Geometry check sheet. Reference: the model listing, model coordinates, mm. Face numbers are marked on the shaded views. A direction names the side the tool comes from. Round coordinates to 2 decimals unless told otherwise and drop trailing zeros. Order: outer loops, then holes, each group sorted by start corner. A loop starts at its lowest first (then second) coordinate and runs counter-clockwise, first axis right, second up.
(1) Release check for a two-part mould opening along X. For the marked faces 4, 5 and 6 record: +X half, -X half, draft (parallel to the pull), parting line (faces both ways), or undercut.
(2) Sectioned sample at C-C (x = 28). Record the boundary of the cut face in (y, z), plus the area to 3 significant figures.
(3) Go/stop test with flat-tipped pins: pin 1 (6.5 mm diameter, centred on x = -3.31, z = 10.66, fed in from +Y); pin 2 (4.5 mm diameter, centred on x = 47.69, z = 17.16, fed in from -Y). Record where each tip stops, or that it passes through.
(4) Set-up check for the marked faces 1, 2 and 3: record each of +Z, -Z, +X, -X, +Y, -Y from which the full face is reachable in a straight line by a thin tool's end or side.
(5) Sectioned sample at D-D (y = -3). Give the number of separate pieces and of enclosed holes in the cut face, plus the area to 3 significant figures.
(6) Material ranges on line 1 along X through (y, z) = (-3.25, 11); line 2 along X through (y, z) = (-2.5, 9.75); line 3 along Z through (x, y) = (30, -3.25), recorded low to high.
(7) Sectioned sample at A-A (x = 0.5). Record the boundary of the cut face in (y, z), plus the area to 3 significant figures.
(8) Sectioned sample at B-B (z = 20). Record the boundary of the cut face in (x, y), plus the area to 3 significant figures.
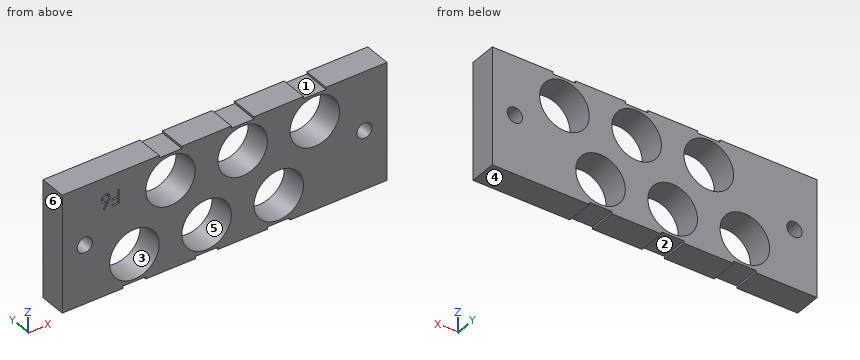
from build123d import *

# Parameters (mm, degrees)
SKETCH1_R               = 5.5
BOSS_EXTRUDE1_DEPTH     = 6
BOSS_EXTRUDE1_2_DEPTH   = 6
BOSS_EXTRUDE1_3_DEPTH   = 6
BOSS_EXTRUDE1_4_DEPTH   = 6
BOSS_EXTRUDE1_5_DEPTH   = 6
BOSS_EXTRUDE1_6_DEPTH   = 6
BOSS_EXTRUDE2_START     = -6
BOSS_EXTRUDE2_OUTLINE_R = 1.7
BOSS_EXTRUDE2_DEPTH     = 6
CUT_EXTRUDE1_DEPTH      = 1


# Read off the part's stored shape, not the designer's step: Boss-Extrude2
with BuildPart() as part:
    # Sketch1 → Boss-Extrude1 (new body)
    with BuildSketch(Plane(origin=(0, 0, 0), x_dir=(1, 0, 0), z_dir=(0, 1, 0))):
        Polygon((2.686395113, -16.66487452), (2.68639507, -4.66487452), (-9.31360493, -4.664874562), (-9.313604887, -16.664874562), align=None)
        with Locations(Location((-3.313604908, -10.664874541, 0), (0, 0, 270))):
            Circle(SKETCH1_R, mode=Mode.SUBTRACT)
    extrude(amount=-BOSS_EXTRUDE1_DEPTH)



with BuildPart() as body_2:
    # Sketch1 → Boss-Extrude1 2 (new body)
    with BuildSketch(Plane(origin=(0, 0, 0), x_dir=(1, 0, 0), z_dir=(0, 1, 0))):
        Polygon((18.686395113, -16.664873819), (18.68639507, -4.664873819), (6.68639507, -4.664873862), (6.686395113, -16.664873862), align=None)
        with Locations(Location((12.686395092, -10.66487384, 0), (0, 0, 270))):
            Circle(SKETCH1_R, mode=Mode.SUBTRACT)
    extrude(amount=-BOSS_EXTRUDE1_2_DEPTH)


with BuildPart() as body_3:
    # Sketch1 → Boss-Extrude1 3 (new body)
    with BuildSketch(Plane(origin=(0, 0, 0), x_dir=(1, 0, 0), z_dir=(0, 1, 0))):
        Polygon((34.686395113, -16.664873762), (34.68639507, -4.664873762), (22.68639507, -4.664873805), (22.686395113, -16.664873805), align=None)
        with Locations(Location((28.686395092, -10.664873784, 0), (0, 0, 270))):
            Circle(SKETCH1_R, mode=Mode.SUBTRACT)
    extrude(amount=-BOSS_EXTRUDE1_3_DEPTH)


with BuildPart() as body_4:
    # Sketch1 → Boss-Extrude1 4 (new body)
    with BuildSketch(Plane(origin=(0, 0, 0), x_dir=(1, 0, 0), z_dir=(0, 1, 0))):
        Polygon((14.68639512, -17.664873833), (14.686395163, -29.664873833), (26.686395163, -29.664873791), (26.68639512, -17.664873791), align=None)
        with Locations(Location((20.686395141, -23.664873812, 0), (0, 0, 270))):
            Circle(SKETCH1_R, mode=Mode.SUBTRACT)
    extrude(amount=-BOSS_EXTRUDE1_4_DEPTH)


with BuildPart() as body_5:
    # Sketch1 → Boss-Extrude1 5 (new body)
    with BuildSketch(Plane(origin=(0, 0, 0), x_dir=(1, 0, 0), z_dir=(0, 1, 0))):
        Polygon((-1.31360488, -17.664873456), (-1.313604837, -29.664873456), (10.686395163, -29.664873413), (10.68639512, -17.664873413), align=None)
        with Locations(Location((4.686395141, -23.664873434, 0), (0, 0, 270))):
            Circle(SKETCH1_R, mode=Mode.SUBTRACT)
    extrude(amount=-BOSS_EXTRUDE1_5_DEPTH)


with BuildPart() as body_6:
    # Sketch1 → Boss-Extrude1 6 (new body)
    with BuildSketch(Plane(origin=(0, 0, 0), x_dir=(1, 0, 0), z_dir=(0, 1, 0))):
        Polygon((30.68639512, -17.664873979), (30.686395163, -29.664873979), (42.686395163, -29.664873936), (42.68639512, -17.664873936), align=None)
        with Locations(Location((36.686395141, -23.664873958, 0), (0, 0, 270))):
            Circle(SKETCH1_R, mode=Mode.SUBTRACT)
    extrude(amount=-BOSS_EXTRUDE1_6_DEPTH)


with BuildPart() as part_1:
    add(part.part)

    add(body_2.part)  # Boss-Extrude2 merges body 2

    add(body_3.part)  # Boss-Extrude2 merges body 3

    add(body_4.part)  # Boss-Extrude2 merges body 4

    add(body_5.part)  # Boss-Extrude2 merges body 5

    add(body_6.part)  # Boss-Extrude2 merges body 6
    # Boss-Extrude2 outline → Boss-Extrude2 (add)
    with BuildSketch(Plane(origin=(0, 0, 0), x_dir=(1, 0, 0), z_dir=(0, 1, 0)).offset(BOSS_EXTRUDE2_START)):
        Polygon((10.186395069, -4.164873849), (-0.813604931, -4.164873888), (-0.81360493, -4.664874532), (2.68639507, -4.66487452), (2.686395113, -16.66487452), (-9.313604887, -16.664874562), (-9.31360493, -4.664874562), (-5.81360493, -4.66487455), (-5.813604931, -4.16487455), (-19.313604998, -4.164874546), (-19.313604998, -30.16487344), (2.186395164, -30.164873443), (2.186395163, -29.664873443), (-1.313604837, -29.664873456), (-1.31360488, -17.664873456), (10.68639512, -17.664873413), (10.686395163, -29.664873413), (7.186395163, -29.664873426), (7.186395164, -30.164873425), (18.186395164, -30.164873821), (18.186395163, -29.664873821), (14.686395163, -29.664873833), (14.68639512, -17.664873833), (26.68639512, -17.664873791), (26.686395163, -29.664873791), (23.186395163, -29.664873803), (23.186395164, -30.164873803), (34.186395164, -30.164873764), (34.186395163, -29.664873966), (30.686395163, -29.664873979), (30.68639512, -17.664873979), (42.68639512, -17.664873936), (42.686395163, -29.664873936), (39.186395163, -29.664873949), (39.186395164, -30.164873949), (52.686395098, -30.16487344), (52.686395098, -4.164874546), (31.186395069, -4.164873775), (31.18639507, -4.664873775), (34.68639507, -4.664873762), (34.686395113, -16.664873762), (22.686395113, -16.664873805), (22.68639507, -4.664873805), (26.18639507, -4.664873792), (26.186395069, -4.164873793), (15.186395069, -4.164873832), (15.18639507, -4.664873832), (18.68639507, -4.664873819), (18.686395113, -16.664873819), (6.686395113, -16.664873862), (6.68639507, -4.664873862), (10.18639507, -4.664873849), align=None)
        with Locations((-14.313604998, -17.164873993)):
            Circle(BOSS_EXTRUDE2_OUTLINE_R, mode=Mode.SUBTRACT)
        with Locations((47.686395098, -17.164873993)):
            Circle(BOSS_EXTRUDE2_OUTLINE_R, mode=Mode.SUBTRACT)
    extrude(amount=BOSS_EXTRUDE2_DEPTH)

    # Sketch2 → Cut-Extrude1 (cut)
    # profile 1 of 2: a face of its own
    with BuildSketch(Plane(origin=(0, -6, 0), x_dir=(-1, 0, 0), z_dir=(0, -1, 0))):
        Polygon((6.699801581, -23.2390136), (8.246596453, -23.2390136), (8.246596453, -23.564654626), (6.984737478, -23.564654626), (6.984737478, -24.541577703), (8.246596453, -24.541577703), (8.246596453, -24.867218728), (6.984737478, -24.867218728), (6.984737478, -26.4140136), (6.699801581, -26.4140136), align=None)
    # profile 2 of 2: a face of its own
    with BuildSketch(Plane(origin=(0, -6, 0), x_dir=(-1, 0, 0), z_dir=(0, -1, 0))):
        with BuildLine():
            Line((9.996916965, -23.157603344), (10.216979065, -23.329964121))
            Line((10.216979065, -23.329964121), (9.378071813, -24.612811677))
            add(Edge.make_bspline(
                [(9.378071813, -24.612811677), (9.43392485, -24.603909103), (9.542872514, -24.586543627), (9.65315015, -24.583678919), (9.706892927, -24.582282831)],
                knots=[0, 0, 0, 0, 1.025318673, 2, 2, 2, 2], degree=3))
            add(Edge.make_bspline(
                [(9.706892927, -24.582282831), (9.739163887, -24.583137599), (9.802478203, -24.584814619), (9.895509725, -24.598067595), (9.984924431, -24.618695779), (10.070522851, -24.64888638), (10.152413619, -24.68743998), (10.231065003, -24.733649384), (10.30499899, -24.789897237), (10.375167554, -24.852730491), (10.438873565, -24.922323744), (10.49527613, -24.996166388), (10.542653291, -25.074181472), (10.581092491, -25.156329486), (10.610941917, -25.2424838), (10.632702138, -25.332534184), (10.645565054, -25.426542733), (10.647311749, -25.490476506), (10.648199017, -25.522952903)],
                knots=[0, 0, 0, 0, 1.044136307, 2.048553127, 3.035567123, 4.010001674, 4.980053131, 5.96154148, 6.956538004, 7.981742224, 9.006487041, 10.005615874, 10.984750588, 11.954802044, 12.935714515, 13.930994945, 14.949008866, 16, 16, 16, 16], degree=3))
            add(Edge.make_bspline(
                [(10.648199017, -25.522952903), (10.646908057, -25.567384491), (10.644367755, -25.654815343), (10.619055025, -25.782157069), (10.579721633, -25.903471565), (10.523499161, -26.016821942), (10.453665142, -26.122052845), (10.368504755, -26.215293946), (10.271038162, -26.298451765), (10.160832281, -26.36799027), (10.042229735, -26.42478018), (9.917631851, -26.465570078), (9.788248654, -26.49068294), (9.700433045, -26.493831272), (9.656011517, -26.495423856)],
                knots=[0, 0, 0, 0, 1.031375318, 2.029502543, 3.004789286, 3.987476834, 4.960371455, 5.9300674, 6.912260825, 7.929083631, 8.949397511, 9.960523116, 10.96833055, 12, 12, 12, 12], degree=3))
            add(Edge.make_bspline(
                [(9.656011517, -26.495423856), (9.613288081, -26.494037555), (9.528660436, -26.491291536), (9.404170686, -26.466829578), (9.284552092, -26.427180992), (9.170642725, -26.372558039), (9.065123312, -26.303562674), (8.970720913, -26.220502607), (8.887906232, -26.125153306), (8.818986397, -26.017529563), (8.764323119, -25.901877958), (8.723329401, -25.781284966), (8.699384238, -25.656189983), (8.69603819, -25.571389235), (8.694352863, -25.528677062)],
                knots=[0, 0, 0, 0, 1.012016664, 2.004627821, 2.994792927, 3.992885782, 4.990978636, 5.973936114, 6.964471063, 7.975201453, 8.993600317, 9.990122807, 10.98767138, 12, 12, 12, 12], degree=3))
            add(Edge.make_bspline(
                [(8.694352863, -25.528677062), (8.695424602, -25.495979475), (8.697612889, -25.429217252), (8.712892251, -25.328103455), (8.737443886, -25.224642831), (8.764939609, -25.136872955), (8.793991413, -25.064971432), (8.818169074, -25.007001837), (8.848262627, -24.947347149), (8.880351337, -24.883961779), (8.91732364, -24.818479279), (8.957524265, -24.749805236), (9.002064662, -24.679031831), (9.033288667, -24.631003882), (9.049250699, -24.606451501)],
                knots=[0, 0, 0, 0, 1.173818275, 2.396712641, 3.66331629, 4.989737886, 5.693666774, 6.447286557, 7.243889047, 8.091586357, 8.998013824, 9.943181721, 10.948533338, 12, 12, 12, 12], degree=3))
            Line((9.049250699, -24.606451501), (9.996916965, -23.157603344))
        make_face()
        with BuildLine():
            add(Edge.make_bspline(
                [(9.64710727, -24.907923856), (9.622921579, -24.908639019), (9.575469451, -24.910042162), (9.505937895, -24.917966716), (9.440309411, -24.932982832), (9.377830069, -24.952402516), (9.31916676, -24.978858553), (9.263592246, -25.010560401), (9.211746157, -25.048541998), (9.16388158, -25.091418934), (9.120507249, -25.138406483), (9.083148796, -25.188723076), (9.050925237, -25.241169384), (9.024725214, -25.296180139), (9.004323526, -25.353735218), (8.989565892, -25.413569669), (8.981352848, -25.476084793), (8.97998648, -25.518477849), (8.97928876, -25.540125379)],
                knots=[0, 0, 0, 0, 1.128956033, 2.215002439, 3.259141796, 4.2666399, 5.263148119, 6.255916712, 7.247353359, 8.256307737, 9.250603402, 10.226115518, 11.176314381, 12.118911324, 13.063945463, 14.021379252, 14.989639887, 16, 16, 16, 16], degree=3))
            add(Edge.make_bspline(
                [(8.97928876, -25.540125379), (8.97985696, -25.561579289), (8.980971114, -25.603647213), (8.991087861, -25.665640612), (9.006541115, -25.725298779), (9.029528474, -25.782314158), (9.056948579, -25.837555818), (9.093148409, -25.889022827), (9.133259351, -25.939841033), (9.181205419, -25.986106654), (9.232661612, -26.029156591), (9.28763556, -26.066785107), (9.344930667, -26.098976136), (9.405320457, -26.124204774), (9.467948134, -26.144909663), (9.533335493, -26.159479719), (9.601528012, -26.167717054), (9.647721485, -26.169085201), (9.67127594, -26.169782831)],
                knots=[0, 0, 0, 0, 0.989467248, 1.94019797, 2.891935182, 3.827694429, 4.772920941, 5.730924762, 6.725747692, 7.756678648, 8.79901574, 9.819492441, 10.826891316, 11.826466727, 12.835195252, 13.867842842, 14.912794438, 16, 16, 16, 16], degree=3))
            add(Edge.make_bspline(
                [(9.67127594, -26.169782831), (9.694830356, -26.169085146), (9.741023753, -26.167716892), (9.809216821, -26.159480335), (9.874602152, -26.144907404), (9.9372372, -26.124212963), (9.997599783, -26.09894576), (10.054844781, -26.066985375), (10.109298837, -26.028925183), (10.16078881, -25.986180223), (10.208535311, -25.939577707), (10.249608271, -25.889476459), (10.28469949, -25.837139854), (10.313214788, -25.782531768), (10.335948959, -25.725264304), (10.351480576, -25.665649848), (10.361576431, -25.603644795), (10.362693456, -25.561578473), (10.363263119, -25.540125379)],
                knots=[0, 0, 0, 0, 1.087397944, 2.132534446, 3.165364764, 4.174271784, 5.174024072, 6.181601208, 7.194203697, 8.236725232, 9.267838612, 10.269026844, 11.221737037, 12.171628256, 13.107553087, 14.05945871, 15.010357665, 16, 16, 16, 16], degree=3))
            add(Edge.make_bspline(
                [(10.363263119, -25.540125379), (10.362763924, -25.518449609), (10.361784167, -25.475907121), (10.350702565, -25.413597625), (10.335333378, -25.35343124), (10.31212604, -25.29578579), (10.28197527, -25.240889945), (10.245252874, -25.18846183), (10.202761835, -25.138117296), (10.153715725, -25.091298499), (10.100325283, -25.048806355), (10.043918117, -25.010417813), (9.98414317, -24.979153645), (9.922078942, -24.95231253), (9.856977887, -24.933290658), (9.789551091, -24.917919833), (9.719159645, -24.910108409), (9.671290808, -24.908657076), (9.64710727, -24.907923856)],
                knots=[0, 0, 0, 0, 0.978753431, 1.920974676, 2.853199117, 3.782215702, 4.721507756, 5.67862441, 6.671401678, 7.694929396, 8.738190014, 9.75360867, 10.774035531, 11.783329636, 12.805060902, 13.835252836, 14.906360638, 16, 16, 16, 16], degree=3))
        make_face(mode=Mode.SUBTRACT)
    extrude(amount=-CUT_EXTRUDE1_DEPTH, mode=Mode.SUBTRACT)


solid = part_1.part
Answer below:
1. face 4: draft
1. face 5: undercut
1. face 6: -X half
2. outline: (-6, 4.66) - (0, 4.66) - (0, 5.21) - (-6, 5.21) - close; (-6, 16.12) - (0, 16.12) - (0, 30.16) - (-6, 30.16) - close
2. area: 87.5 mm2
3. pin 1: passes through
3. pin 2: stops at y = -6
4. face 1: +Z, +Y, -Y
4. face 2: -Z, +Y, -Y
4. face 3: +Y, -Y
5. separate pieces: 1
5. enclosed holes: 8
5. area: 1,270 mm2
6. line 1: x = -19.31 to -8.8, 2.18 to 7.2, 18.18 to 23.2, 34.18 to 52.69
6. line 2: x = -19.31 to -8.74, 2.11 to 7.26, 18.11 to 23.26, 34.11 to 52.69
6. line 3: z = 4.66 to 5.32, 16.01 to 30.16
7. outline: (-6, 4.16) - (0, 4.16) - (0, 6.7) - (-6, 6.7) - close; (-6, 14.63) - (0, 14.63) - (0, 20.1) - (-6, 20.1) - close; (-6, 27.23) - (0, 27.23) - (0, 30.16) - (-6, 30.16) - close
7. area: 65.6 mm2
8. outline: (-19.31, -6) - (0.59, -6) - (0.59, 0) - (-19.31, 0) - close; (8.79, -6) - (16.59, -6) - (16.59, 0) - (8.79, 0) - close; (24.79, -6) - (32.59, -6) - (32.59, 0) - (24.79, 0) - close; (40.79, -6) - (52.69, -6) - (52.69, 0) - (40.79, 0) - close
8. area: 284 mm2
